Input: part model. Units: mm. Frame: model coordinates. Face numbers are marked on the shaded views. A direction names the side the tool comes from. Round coordinates to 2 decimals unless told otherwise and drop trailing zeros. Order: outer loops, then holes, each group sorted by start corner. A loop starts at its lowest first (then second) coordinate and runs counter-clockwise, first axis right, second up. Notation, with made-up numbers: (30, -34) -> (39, -34) arc R25 ccw to (39, -11) -> close; hole circle Ø9 at (17.5, -5). An arc over 180 degrees is marked (long way). Use a Markdown table: item, result.
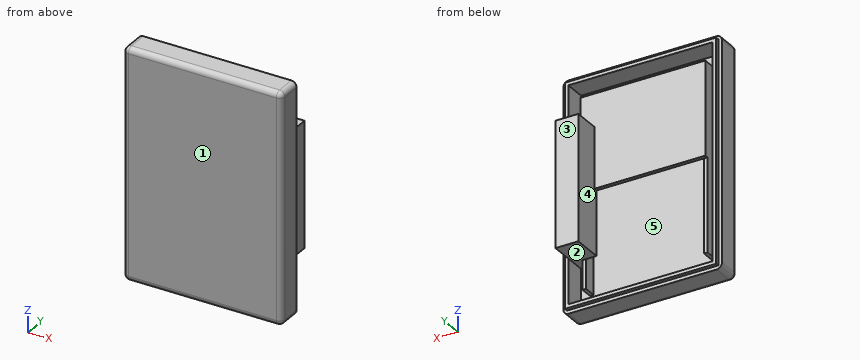
Autodesk Inventor part; units mm, degrees
ref_plane "YZ Plane" through (0, 0, 0) normal (1, 0, 0) x (0, 1, 0)
ref_plane "XZ Plane" through (0, 0, 0) normal (0, 1, 0) x (-1, 0, 0)
ref_plane "XY Plane" through (0, 0, 0) normal (0, 0, 1) x (1, 0, 0)
sketch "Sketch1" plane through (0, 0, 0) normal (0, 1, 0) x (-1, 0, 0)
  line L0 (0, 0) -> (45, 0)
  line L1 (45, 0) -> (45, -65)
  line L2 (45, -65) -> (0, -65)
  line L3 (0, -65) -> (0, 0)
  dimension "d0" = 45
  dimension "d1" = 65
extrude "Extrusion1" add sketch "Sketch1" along normal blind 2
sketch "Sketch2" plane through (0, 2, 0) normal (0, 1, 0) x (1, 0, 0)
  line L0 (0, 65) -> (0, 0)
  line L1 (0, 0) -> (-45, 0)
  line L2 (-45, 0) -> (-45, 65)
  line L3 (-45, 65) -> (0, 65)
  line L4 (-45, 0) -> (0, 0)
  line L5 (-45, 65) -> (-45, 0)
  line L6 (0, 65) -> (-45, 65)
  line L7 (0, 0) -> (0, 65)
  line L8 (-2, 2) -> (-43, 2)
  line L9 (-43, 2) -> (-43, 63)
  line L10 (-43, 63) -> (-2, 63)
  line L11 (-2, 63) -> (-2, 2)
  dimension "d4" = 2
  dimension "d5" = 2
  dimension "d6" = 2
  dimension "d7" = 2
extrude "Extrusion2" add sketch "Sketch2" along normal blind 2
sketch "Sketch3" plane through (0, 2, 0) normal (0, 1, 0) x (1, 0, 0)
  line L0 (-5.5, 6.5) -> (-39, 6.5)
  line L1 (-39, 6.5) -> (-39, 57.5)
  line L2 (-39, 57.5) -> (-5.5, 57.5)
  line L3 (-5.5, 57.5) -> (-5.5, 6.5)
  line L4 (0, 0) -> (0, 65) construction
  line L5 (0, 32.5) -> (-39, 32.5) construction
  line L6 (-45, 0) -> (0, 0) construction
  line L7 (-22.5, 0) -> (-22.5, 65) construction
  line L8 (0, 65) -> (-45, 65) construction
  line L9 (-4.5, 58.5) -> (-40, 58.5)
  line L10 (-40, 58.5) -> (-40, 5.5)
  line L11 (-40, 5.5) -> (-4.5, 5.5)
  line L12 (-4.5, 5.5) -> (-4.5, 58.5)
  line L13 (-2, 2) -> (-2, 63)
  line L14 (-2, 63) -> (-43, 63)
  line L15 (-43, 63) -> (-43, 2)
  line L16 (-43, 2) -> (-2, 2)
  line L17 (0, 65) -> (0, 0)
  line L18 (0, 0) -> (-45, 0)
  line L19 (-45, 0) -> (-45, 65)
  line L20 (-45, 65) -> (0, 65)
  dimension "d10" = 33.5
  dimension "d11" = 51
  dimension "d12" = 26
  dimension "d13" = 17
  dimension "d14" = 1
  dimension "d15" = 1
  dimension "d16" = 1
  dimension "d17" = 1
  dimension "d25" = 51
extrude "Extrusion3" add sketch "Sketch3" along normal blind 3.5 contours L12 L11 L10 L9
sketch "Sketch4" plane through (-4.5, 2, -58.5) normal (0, 0, -1) x (-1, 0, 0)
  line L0 (35.5, 0) -> (0, 0)
  line L1 (35.5, 0) -> (35.5, 3.5)
  line L2 (0, 3.5) -> (35.5, 3.5)
  line L3 (0, 0) -> (0, 3.5)
  line L4 (1, 3.5) -> (34.5, 3.5)
  line L5 (34.5, 3.5) -> (34.5, 0)
  line L6 (34.5, 0) -> (1, 0)
  line L7 (1, 0) -> (1, 3.5)
  point P0 (-4.5, -2)
  point P1 (1, 0)
  point P2 (34.5, 0)
  dimension "d20" = 1
  dimension "d21" = 1
  dimension "d22" = 0
extrude "Extrusion4" cut sketch "Sketch4" against normal blind 2 contours L0 L7 L2 L5
sketch "Sketch5" plane through (0, 5.5, 0) normal (0, 1, 0) x (1, 0, 0)
  line L0 (-39, 58.5) -> (-39, 6.5)
  line L1 (-39, 6.5) -> (-5.5, 6.5)
  line L2 (-5.5, 6.5) -> (-5.5, 58.5)
  line L3 (-5.5, 58.5) -> (-4.5, 58.5)
  line L4 (-4.5, 58.5) -> (-4.5, 5.5)
  line L5 (-4.5, 5.5) -> (-40, 5.5)
  line L6 (-40, 5.5) -> (-40, 58.5)
  line L7 (-40, 58.5) -> (-39, 58.5)
  line L8 (-40, 5.5) -> (-4.5, 5.5)
  line L9 (-4.5, 5.5) -> (-4.5, 32)
  line L10 (-4.5, 32) -> (-40, 32)
  line L11 (-40, 32.75) -> (-40, 5.5)
  line L12 (-4.5, 32) -> (-40, 32)
  line L13 (-40, 32) -> (-40, 5.5)
  line L14 (-40, 5.5) -> (-4.5, 5.5)
  line L15 (-4.5, 5.5) -> (-4.5, 32)
  line L16 (-40, 58.5) -> (-40, 5.5)
  line L17 (-40, 5.5) -> (-4.5, 5.5)
  line L18 (-4.5, 5.5) -> (-4.5, 58.5)
  line L19 (-4.5, 32) -> (-40, 32)
  line L20 (-40, 32) -> (-40, 5.5)
  line L21 (-40, 5.5) -> (-4.5, 5.5)
  line L22 (-4.5, 5.5) -> (-4.5, 32.75)
  point P0 (0, 0)
  point P1 (-5.5, 32)
  point P2 (-39, 32)
extrude "Extrusion6" add sketch "Sketch5" along normal blind 1 contours L10 L2 L1 L0 | L0 L1 L2 L10 L4 L5 L6
fillet "Fillet1" radius 1.5 1 edges at (-22.5, 0, 0)
fillet "Fillet2" radius 1.5 1 edges at (-22.5, 0, -65)
sketch "Sketch13" plane through (0, 6.5, 0) normal (0, 1, 0) x (1, 0, 0)
  line L0 (0, 0) -> (0, 65)
  line L1 (-4.5, 5.5) -> (-4.5, 32)
  line L2 (-4.5, 32) -> (-4.5, 58.5)
  line L3 (-5.5, 6.5) -> (-5.5, 58.5)
  line L4 (-40, 32) -> (-40, 5.5) construction
  line L5 (-40, 5.5) -> (-4.5, 5.5) construction
  line L6 (-4.5, 5.5) -> (-4.5, 32) construction
  line L7 (-4.5, 32) -> (-40, 32) construction
  line L8 (-2, 63) -> (-2, 2)
  line L9 (-40, 5.5) -> (-4.5, 5.5)
  line L10 (-4.5, 32) -> (-40, 32)
  line L11 (-2, 50.25) -> (-8.5, 50.25)
  line L12 (-8.5, 50.25) -> (-8.5, 14.75)
  line L13 (-8.5, 14.75) -> (-2, 14.75)
  line L14 (-2, 14.75) -> (-2, 50.25)
  line L15 (-2, 2) -> (-43, 2)
  point P0 (-5.75, 59.75)
  point P1 (-4.5, 14.75)
  point P2 (-2, 14.75)
  point P3 (-4.5, 50.25)
  dimension "d58" = 6.5
  dimension "d59" = 35.5
  dimension "d60" = 12.75
extrude "Extrusion12" add sketch "Sketch13" along normal mid plane 15
sketch "Sketch14" plane through (-2, -1, -14.75) normal (1, 0, 0) x (0, 0, -1)
  line L0 (0, 0) -> (35.5, 0)
  line L1 (0, 0) -> (0, 1)
  line L2 (35.5, 0) -> (0, 0)
  line L3 (0, 0) -> (0, 1)
  line L4 (0, 1) -> (35.5, 1)
  line L5 (35.5, 1) -> (35.5, 0)
  point P0 (-14.75, 1)
extrude "Extrusion13" cut sketch "Sketch14" against normal through all
sketch "Sketch15" plane through (-2, 14, -50.25) normal (0, 0, -1) x (-1, 0, 0)
  line L0 (6.5, -7.5) -> (38, -7.5)
  line L1 (6.5, -8.5) -> (37, -8.5)
  line L2 (3.5, -12) -> (3.5, -8.5)
  line L3 (37, -12) -> (3.5, -12)
  line L4 (3.5, -8.5) -> (6.5, -8.5)
  line L5 (6.5, -8.5) -> (6.5, -12)
  line L6 (6.5, -12) -> (3.5, -12)
  line L7 (3.5, -12) -> (3.5, -8.5)
  point P0 (-2, -14)
extrude "Extrusion14" cut sketch "Sketch15" against normal up to surface (43.75 mm away)
sketch "Sketch16" plane through (0, 4, 0) normal (0, 1, 0) x (1, 0, 0)
  line L0 (-2, 14.75) -> (-2, 50.25)
  line L1 (-2, 14.75) -> (-2, 2)
  line L2 (-2, 2) -> (-43, 2)
  line L3 (-45, 0) -> (0, 0)
  line L4 (0, 0) -> (0, 65)
  line L5 (-2, 63) -> (-2, 50.25)
  line L6 (-43, 63) -> (-2, 63)
  line L7 (0, 65) -> (-45, 65)
  line L8 (-45, 65) -> (-45, 0)
  line L9 (-43, 2) -> (-43, 63)
  line L10 (0, 65) -> (-45, 65)
  line L11 (-45, 65) -> (-45, 0)
  line L12 (-45, 0) -> (0, 0)
  line L13 (0, 0) -> (0, 65)
  line L14 (-43, 2) -> (-2, 2)
  line L15 (-2, 2) -> (-2, 63)
  line L16 (-2, 63) -> (-43, 63)
  line L17 (-43, 63) -> (-43, 2)
extrude "Extrusion15" add sketch "Sketch16" along normal blind 4
sketch "Sketch17" plane through (0, 8, 0) normal (0, 1, 0) x (1, 0, 0)
  line L0 (0, 0) -> (0, 65)
  line L1 (0, 65) -> (-45, 65)
  line L2 (-45, 0) -> (0, 0)
  line L3 (-45, 65) -> (-45, 0)
  line L4 (-1, 64) -> (-44, 64)
  line L5 (-44, 64) -> (-44, 1)
  line L6 (-44, 1) -> (-1, 1)
  line L7 (-1, 1) -> (-1, 64)
  dimension "d71" = 1
  dimension "d72" = 1
  dimension "d73" = 1
  dimension "d74" = 1
extrude "Extrusion16" cut sketch "Sketch17" against normal blind 1
fillet "Fillet3" radius 1.5 5 edges at (0, 0.4393, -0.4393) (0, 0, -32.5) (0, 0.4393, -64.5607) (0, 4.25, -65) (0, 4.25, 0)
fillet "Fillet4" radius 1.5 5 edges at (-45, 0.4393, -0.4393) (-45, 4.25, 0) (-45, 0.4393, -64.5607) (-45, 4.25, -65) (-45, 0, -32.5)
equation "\"BendRadius\" = Thickness"
equation "\"BendReliefWidth\" = Thickness"
equation "\"BendReliefDepth\" = 0.5 * Thickness"
equation "\"CornerReliefSize\" = 4 * Thickness"
equation "\"MinimumRemnant\" = 2 * Thickness"
equation "\"TransitionRadius\" = BendRadius"
equation "\"JacobiRadiusSize\" = BendRadius"
equation "\"GapSize\" = Thickness"
properties part number "superior" material "ABS Plastic"
1) Cut plane D-D on x = -32. Return loops of the section in (y, z).
Results found:
| item | result |
|---|---|
| outline | (0, -63.5) arc R1.5 ccw to (1.5, -65) -> (7, -65) -> (7, -64) -> (8, -64) -> (8, -63) -> (2, -63) -> (2, -6.5) -> (5.5, -6.5) -> (5.5, -32) -> (6.5, -32) -> (6.5, -5.5) -> (2, -5.5) -> (2, -2) -> (8, -2) -> (8, -1) -> (7, -1) -> (7, 0) -> (1.5, 0) arc R1.5 ccw to (0, -1.5) -> close |
2) Pin query (flat end, axial travel): pin 1 Ø1.8 at (x, y) = (-17, 3.5) entering from +Z; pin 2 Ø1 at (x, z) = (-21, -40.5) entering from +Y; pin 3 Ø1.8 at (y, z) = (11.5, -38.5) entering from +X; pin 4 Ø0.5 at (y, z) = (7.5, -45.5) entering from -X. Return the tip coordinate at first contact, or that it passes through.
Results found:
| item | result |
|---|---|
| pin 1 | stops at z = 0 |
| pin 2 | stops at y = 2 |
| pin 3 | stops at x = -2 |
| pin 4 | stops at x = -44 |
3) Cut plane C-C on z = -13. Return loops of the section in (x, y).
Results found:
| item | result |
|---|---|
| outline | (-45, 1.5) arc R1.5 ccw to (-43.5, 0) -> (-1.5, 0) arc R1.5 ccw to (0, 1.5) -> (0, 7) -> (-1, 7) -> (-1, 8) -> (-2, 8) -> (-2, 2) -> (-4.5, 2) -> (-4.5, 6.5) -> (-40, 6.5) -> (-40, 2) -> (-43, 2) -> (-43, 8) -> (-44, 8) -> (-44, 7) -> (-45, 7) -> close; hole (-39, 2) -> (-5.5, 2) -> (-5.5, 5.5) -> (-39, 5.5) -> close |
4) Set-up query: the marked faces 3, 4 and 5. Return all of +Z, -Z, +X, -X, +Y, -Y with unobstructed straight access to the full face (end or side cutting, diameter ignored); none if empty.
Results found:
| item | result |
|---|---|
| face 3 | +Z, -Z, +X, -X, +Y |
| face 4 | +Y |
| face 5 | none |
5) Cut plane B-B on y = 3.25. Return loops of the section in (x, z), and give its area (3 significant figures).
Results found:
| item | result |
|---|---|
| outline | (-45, -63.5) arc R1.5 ccw to (-43.5, -65) -> (-1.5, -65) arc R1.5 ccw to (0, -63.5) -> (0, -1.5) arc R1.5 ccw to (-1.5, 0) -> (-43.5, 0) arc R1.5 ccw to (-45, -1.5) -> close; hole (-43, -63) -> (-2, -63) -> (-2, -50.25) -> (-4.5, -50.25) -> (-4.5, -58.5) -> (-5.5, -58.5) -> (-5.5, -6.5) -> (-39, -6.5) -> (-39, -58.5) -> (-40, -58.5) -> (-40, -5.5) -> (-4.5, -5.5) -> (-4.5, -14.75) -> (-2, -14.75) -> (-2, -2) -> (-43, -2) -> close |
| area | 650 mm² |
6) Pull-direction query (X, two-part tool) for the marked faces 1 and 2; classes: +X half, -X half, draft (parallel to the pull), parting line (faces both ways), or undercut.
Results found:
| item | result |
|---|---|
| face 1 | draft |
| face 2 | undercut |
7) Cut plane A-A on z = -47. Return loops of the section in (x, y), and give its area (3 significant figures).
Results found:
| item | result |
|---|---|
| outline | (-45, 1.5) arc R1.5 ccw to (-43.5, 0) -> (-1.5, 0) arc R1.5 ccw to (0, 1.5) -> (0, 7) -> (-1, 7) -> (-1, 8) -> (-2, 8) -> (-2, 14) -> (-8.5, 14) -> (-8.5, 5.5) -> (-5.5, 5.5) -> (-5.5, 2) -> (-39, 2) -> (-39, 5.5) -> (-40, 5.5) -> (-40, 2) -> (-43, 2) -> (-43, 8) -> (-44, 8) -> (-44, 7) -> (-45, 7) -> close |
| area | 182 mm² |
8) Line query: L1, parallel to Z at x = -24, y = 3; L2, parallel to X at y = 3.25, z = -47.5; L3, parallel to X at y = 7.25, z = -43. Output: solid intervals per line, ascending. Write a range as [from, to].
Results found:
| item | result |
|---|---|
| L1 | z = [-65, -63], [-6.5, -5.5], [-2, 0] |
| L2 | x = [-45, -43], [-40, -39], [-5.5, 0] |
| L3 | x = [-44, -43], [-8.5, -1] |
